```python
from build123d import *

# Parameters (mm, degrees)
F0_R     = 15.5
F1_DEPTH = 50


with BuildPart() as f1:
    # F0 (on Front) → F1 (new body)
    with BuildSketch(Plane.XZ):
        with BuildLine():
            Line((60, 45), (-60, 45))
            Line((-60, 45), (-60, -45))
            ThreePointArc((-60, -45), (0, -43.829965), (60, -45))
            Line((60, -45), (60, 45))
        make_face()
        Circle(F0_R, mode=Mode.SUBTRACT)
    extrude(amount=F1_DEPTH)


solid = f1.part
```
Model file for the job. Use its own axes, mm. Coordinates: 2 decimals unless noted, no trailing zeros. Order: outer loops, then holes, each group sorted by start corner. A loop starts at its lowest first (then second) coordinate and runs counter-clockwise, first axis right, second up. Notation, with made-up numbers: (-22.75, -14) - (3.25, -14) arc R23 cw to (3.25, 8) - close; hole circle Ø5 at (-26.5, 18.5). An arc over 180 degrees is marked (long way). Return JSON: item names as keys, results as strings. Group by question number.
1) Saw through at A-A, the plane x = 0. Write the cut outline in (y, z), plus the area to 3 significant figures.
2) Probe line 1 (Z direction, x = 0, y = -40); line 2 (X direction, y = -31, z = 2); line 3 (Z direction, x = 4.5, y = -9.5). List the from-to ranges inside material, lowest first. Write a range as from..to.
3) Saw through at B-B, the plane y = -31. Write the cut outline in (x, z).
4) Flat gauge pin, fed straight in: P1, Ø5, axis at x = 46.5, y = -39.5, coming from the -Z side. Where does the tip first touch, or does it go through?
5) Mould opens along X. For faces 1 (the cylindrical face through (-0.84, -24.65, -43.83)), 2 (the flat face through (60, -25, -1)), 3 (the cylindrical face through (-2.018, -24.65, 15.368)), 4 (the flat face through (-60, -25, 1)) say: released by +X, released by -X, zero draft, split by the parting line, or undercut.
6) Saw through at C-C, the plane z = 0. Write the cut outline in (x, y).
Values found:
{
 "1": {"outline": "(-50, -43.83) - (0, -43.83) - (0, -15.5) - (-50, -15.5) - close; (-50, 15.5) - (0, 15.5) - (0, 45) - (-50, 45) - close", "area": "2,890 mm²"},
 "2": {"line 1": "z = -43.83..-15.5, 15.5..45", "line 2": "x = -60..-15.37, 15.37..60", "line 3": "z = -43.84..-14.83, 14.83..45"},
 "3": {"outline": "(-60, -45) arc R1539 cw to (60, -45) - (60, 45) - (-60, 45) - close; hole circle Ø31 at (0, 0)"},
 "4": {"P1": "stops at z = -44.61"},
 "5": {"face 1": "undercut", "face 2": "released by +X", "face 3": "undercut", "face 4": "released by -X"},
 "6": {"outline": "(-60, -50) - (-15.5, -50) - (-15.5, 0) - (-60, 0) - close; (15.5, -50) - (60, -50) - (60, 0) - (15.5, 0) - close"}
}
